The model under review builds one solid part; all positions refer to its coordinate system, in mm. Round coordinates to 2 decimals unless told otherwise and drop trailing zeros. Write each loop counter-clockwise with the first axis right and the second up, starting at its lowest first coordinate (ties: lowest second). Pieces come first, ordered by that corner, then holes.
Item 1: Add section A-A (x = 116). Give the boundary of the cut face in (y, z), plus the area to 3 significant figures.
Item 2: Clearance check with a flat-ended pin moving along its axis: pin 1 Ø2 at (y, z) = (1.5, -198) entering from -X. State where the tip first meets the part, or that it passes through.
Item 3: To check wall thickness, follow L1, parallel to X at y = 0.6, z = -103; L2, parallel to X at y = 3, z = -249; L3, parallel to Z at x = 165, y = 1.65. State the ranges of each line that lie inside material, in increasing order.
Item 4: Add section B-B (z = -186). Give the boundary of the cut face in (x, y).
```python
from build123d import *

# Parameters (mm, degrees)
SKETCH2_W           = 355.6
SKETCH2_H           = 304.8
BOSS_EXTRUDE1_DEPTH = 4.4958
CUT_EXTRUDE3_DEPTH  = 6.35


with BuildPart() as part:
    # Sketch2 → Boss-Extrude1 (new body)
    with BuildSketch(Plane(origin=(0, 0, 0), x_dir=(1, 0, 0), z_dir=(0, 1, 0))):
        with Locations((177.8, 152.4)):
            Rectangle(SKETCH2_W, SKETCH2_H)
    extrude(amount=BOSS_EXTRUDE1_DEPTH)

    # Sketch3 → Cut-Extrude3 (cut)
    with BuildSketch(Plane(origin=(0, 4.4958, 0), x_dir=(1, 0, 0), z_dir=(0, 1, 0))):
        Polygon((60.0075, 49.6443), (60.0075, 55.3085), (165.1, 55.3085), (165.1, 59.8043), (58.1533, 59.8043), (58.1533, 139.7), (53.6575, 139.7), (53.6575, 49.6443), align=None)
        Polygon((190.5, 59.8043), (190.5, 55.3085), (295.5925, 55.3085), (295.5925, 49.6443), (301.9425, 49.6443), (301.9425, 139.7), (297.4467, 139.7), (297.4467, 59.8043), align=None)
        Polygon((53.6575, 165.1), (58.1533, 165.1), (58.1533, 244.9957), (165.1, 244.9957), (165.1, 249.4915), (60.0075, 249.4915), (60.0075, 255.1557), (53.6575, 255.1557), align=None)
        Polygon((297.4467, 244.9957), (297.4467, 165.1), (301.9425, 165.1), (301.9425, 255.1557), (295.5925, 255.1557), (295.5925, 249.4915), (190.5, 249.4915), (190.5, 244.9957), align=None)
    extrude(amount=-CUT_EXTRUDE3_DEPTH, mode=Mode.SUBTRACT)


solid = part.part
```
Numbers:
1. outline: (0, -304.8) - (4.5, -304.8) - (4.5, -249.49) - (0, -249.49) - close; (0, -245) - (4.5, -245) - (4.5, -59.8) - (0, -59.8) - close; (0, -55.31) - (4.5, -55.31) - (4.5, 0) - (0, 0) - close
1. area: 1,330 mm2
2. pin 1: stops at x = 0
3. L1: x = 0 to 53.66, 58.15 to 297.45, 301.94 to 355.6
3. L2: x = 0 to 53.66, 165.1 to 190.5, 301.94 to 355.6
3. L3: z = -304.8 to -249.49, -245 to -59.8, -55.31 to 0
4. outline: (0, 0) - (53.66, 0) - (53.66, 4.5) - (0, 4.5) - close; (58.15, 0) - (297.45, 0) - (297.45, 4.5) - (58.15, 4.5) - close; (301.94, 0) - (355.6, 0) - (355.6, 4.5) - (301.94, 4.5) - close
